```python
from build123d import *

# Parameters (mm, degrees)
SALIENTE_EXTRUIR1_DEPTH = 6
CROQUIS2_R              = 1.75
CORTAR_EXTRUIR1_DEPTH   = 6
CORTAR_EXTRUIR2_DEPTH   = 67.977608199
REDONDEO1_R             = 0.2
REDONDEO2_R             = 2


with BuildPart() as part:
    # Croquis1 → Saliente-Extruir1 (new body)
    with BuildSketch(Plane(origin=(0, 0, 0), x_dir=(1, 0, 0), z_dir=(0, 1, 0))):
        with BuildLine():
            Line((-5, 32.5), (5, 32.5))
            Line((5, 32.5), (15, 32.5))
            Line((15, 32.5), (15, 23.5))
            Line((15, 23.5), (14, 23.5))
            ThreePointArc((14, 23.5), (7.636038969, 20.863961031), (5, 14.5))
            Line((5, 14.5), (5, -14.5))
            ThreePointArc((5, -14.5), (7.636038969, -20.863961031), (14, -23.5))
            Line((14, -23.5), (15, -23.5))
            Line((15, -23.5), (15, -32.5))
            Line((15, -32.5), (5, -32.5))
            Line((5, -32.5), (-5, -32.5))
            Line((-5, -32.5), (-5, 32.5))
        make_face()
    extrude(amount=SALIENTE_EXTRUIR1_DEPTH)

    # Croquis2 → Cortar-Extruir1 (cut)
    with BuildSketch(Plane(origin=(0, 6, 0), x_dir=(1, 0, 0), z_dir=(0, 1, 0))):
        with Locations(Location((10, -28, 0), (0, 0, 270))):
            Circle(CROQUIS2_R)
        with Locations(Location((10, 28, 0), (0, 0, 90))):
            Circle(CROQUIS2_R)
    extrude(amount=-CORTAR_EXTRUIR1_DEPTH, mode=Mode.SUBTRACT)

    # Croquis4 → Cortar-Extruir2 (cut, through all)
    with BuildSketch(Plane.XY.offset(32.5)):
        Polygon((-5, 0), (-1, 0), (-1, 2), (-3, 2), (-3, 1.05), (-5, 1.05), align=None)
        Polygon((-5, 6), (-1, 6), (-1, 4), (-3, 4), (-3, 4.95), (-5, 4.95), align=None)
    extrude(amount=-CORTAR_EXTRUIR2_DEPTH, mode=Mode.SUBTRACT)

    # Redondeo1
    redondeo1_edges = [part.edges().sort_by_distance(p)[0] for p in [
        (-5, 1.05, 0),
        (-3, 1.05, 0),
        (-3, 2, 0),
        (-1, 2, 0),
        (-5, 4.95, 0),
        (-1, 4, 0),
        (-3, 4, 0),
        (-3, 4.95, 0),
    ]]
    fillet(redondeo1_edges, radius=REDONDEO1_R)

    # Redondeo2
    redondeo2_edges = [part.edges().sort_by_distance(p)[0] for p in [
        (15, 3, 32.5),
        (15, 3, 23.5),
        (15, 3, -23.5),
        (15, 3, -32.5),
    ]]
    fillet(redondeo2_edges, radius=REDONDEO2_R)


solid = part.part
```
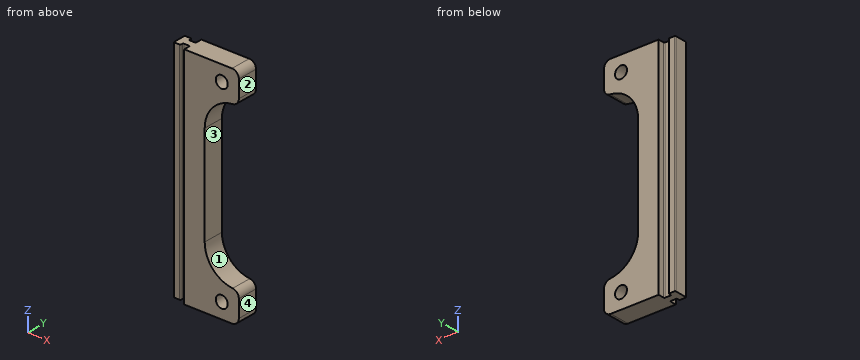
Verification items for the finished model (mm, model axes). Face numbers are marked on the shaded views. A direction names the side the tool comes from. Round coordinates to 2 decimals unless told otherwise and drop trailing zeros. Order: outer loops, then holes, each group sorted by start corner. A loop starts at its lowest first (then second) coordinate and runs counter-clockwise, first axis right, second up. Notation, with made-up numbers: (33.25, -27.75) - (83.25, -27.75) arc R24 cw to (83.25, -11.75) - close; hole circle Ø6 at (-3, 77). An arc over 180 degrees is marked (long way). Use CSV: the item, a comma, the result in double quotes. Start each with the question number.
1) Go/stop test with flat-tipped pins: P1, Ø1.3, axis at x = -2, z = 3, coming from the +Y side; P2, Ø2, axis at x = 10, z = -28, coming from the -Y side; P3, Ø0.5, axis at x = -4, z = -12.5, coming from the +Y side; P4, Ø1.8, axis at x = -4, z = -6, coming from the -Y side. Record where each tip stops, or that it passes through.
2) Section check D-D, the plane z = -21. Record the cut outline in (x, y).
3) Section check A-A, the plane z = -28. Record the cut outline in (x, y), plus the area to 3 significant figures.
4) Mould release check, pull along Z, two halves, no side actions. Record for the marked faces 3 and 4: +Z half, -Z half, draft (parallel to the pull), parting line (faces both ways), or undercut.
5) Section check B-B, the plane x = 10. Record the cut outline in (y, z).
6) Thickness scan on L1, parallel to X at y = 1.35, z = 28; L2, parallel to X at y = 1.5, z = -13; L3, parallel to X at y = 2.75, z = -28. Record the ranges inside material, lowest first.
7) Section check C-C, the plane z = 0. Record the cut outline in (x, y).
8) Access from +Z, -Z, +X, -X, +Y, -Y to the whole of each face (thin tool, end or side, straight path). Record for the marked faces 1 and 2.
Answers:
1,P1,"stops at y = 4"
1,P2,"passes through"
1,P3,"stops at y = 4.95"
1,P4,"stops at y = 1.05"
2,outline,"(-5, 1.25) arc R0.2 ccw to (-4.8, 1.05) - (-3.2, 1.05) arc R0.2 ccw to (-3, 1.25) - (-3, 1.8) arc R0.2 cw to (-2.8, 2) - (-1.2, 2) arc R0.2 cw to (-1, 1.8) - (-1, 0) - (7.78, 0) - (7.78, 6) - (-1, 6) - (-1, 4.2) arc R0.2 cw to (-1.2, 4) - (-2.8, 4) arc R0.2 cw to (-3, 4.2) - (-3, 4.75) arc R0.2 ccw to (-3.2, 4.95) - (-4.8, 4.95) arc R0.2 ccw to (-5, 4.75) - close"
3,outline,"(-5, 1.25) arc R0.2 ccw to (-4.8, 1.05) - (-3.2, 1.05) arc R0.2 ccw to (-3, 1.25) - (-3, 1.8) arc R0.2 cw to (-2.8, 2) - (-1.2, 2) arc R0.2 cw to (-1, 1.8) - (-1, 0) - (8.25, 0) - (8.25, 6) - (-1, 6) - (-1, 4.2) arc R0.2 cw to (-1.2, 4) - (-2.8, 4) arc R0.2 cw to (-3, 4.2) - (-3, 4.75) arc R0.2 ccw to (-3.2, 4.95) - (-4.8, 4.95) arc R0.2 ccw to (-5, 4.75) - close; (11.75, 0) - (15, 0) - (15, 6) - (11.75, 6) - close"
3,area,"86.8 mm²"
4,face 3,"undercut"
4,face 4,"draft"
5,outline,"(0, -32.5) - (6, -32.5) - (6, -29.75) - (0, -29.75) - close; (0, -26.25) - (6, -26.25) - (6, -22.56) - (0, -22.56) - close; (0, 22.56) - (6, 22.56) - (6, 26.25) - (0, 26.25) - close; (0, 29.75) - (6, 29.75) - (6, 32.5) - (0, 32.5) - close"
6,L1,"x = -5 to -3, -1 to 8.25, 11.75 to 15"
6,L2,"x = -5 to -3, -1 to 5"
6,L3,"x = -5 to 8.25, 11.75 to 15"
7,outline,"(-5, 1.25) arc R0.2 ccw to (-4.8, 1.05) - (-3.2, 1.05) arc R0.2 ccw to (-3, 1.25) - (-3, 1.8) arc R0.2 cw to (-2.8, 2) - (-1.2, 2) arc R0.2 cw to (-1, 1.8) - (-1, 0) - (5, 0) - (5, 6) - (-1, 6) - (-1, 4.2) arc R0.2 cw to (-1.2, 4) - (-2.8, 4) arc R0.2 cw to (-3, 4.2) - (-3, 4.75) arc R0.2 ccw to (-3.2, 4.95) - (-4.8, 4.95) arc R0.2 ccw to (-5, 4.75) - close"
8,face 1,"+X, +Y, -Y"
8,face 2,"+Z, -Z, +X, +Y, -Y"
